Job drawing, mm, ordinate dimensions from the low corner. One solid piece. Give positions to 0.01 mm unless a question says otherwise; leave off trailing zeros. Loops run counter-clockwise (first coordinate to the right, second up) from the corner with the lowest first, then second, coordinate; pieces in that order, holes last. Notation, with made-up numbers: (87.25, 54) - (96.25, 54) arc R34 ccw to (96.25, 93) - close; hole circle Ø11 at (25.5, 38). An arc over 180 degrees is marked (long way). Use a Markdown table: item, result.
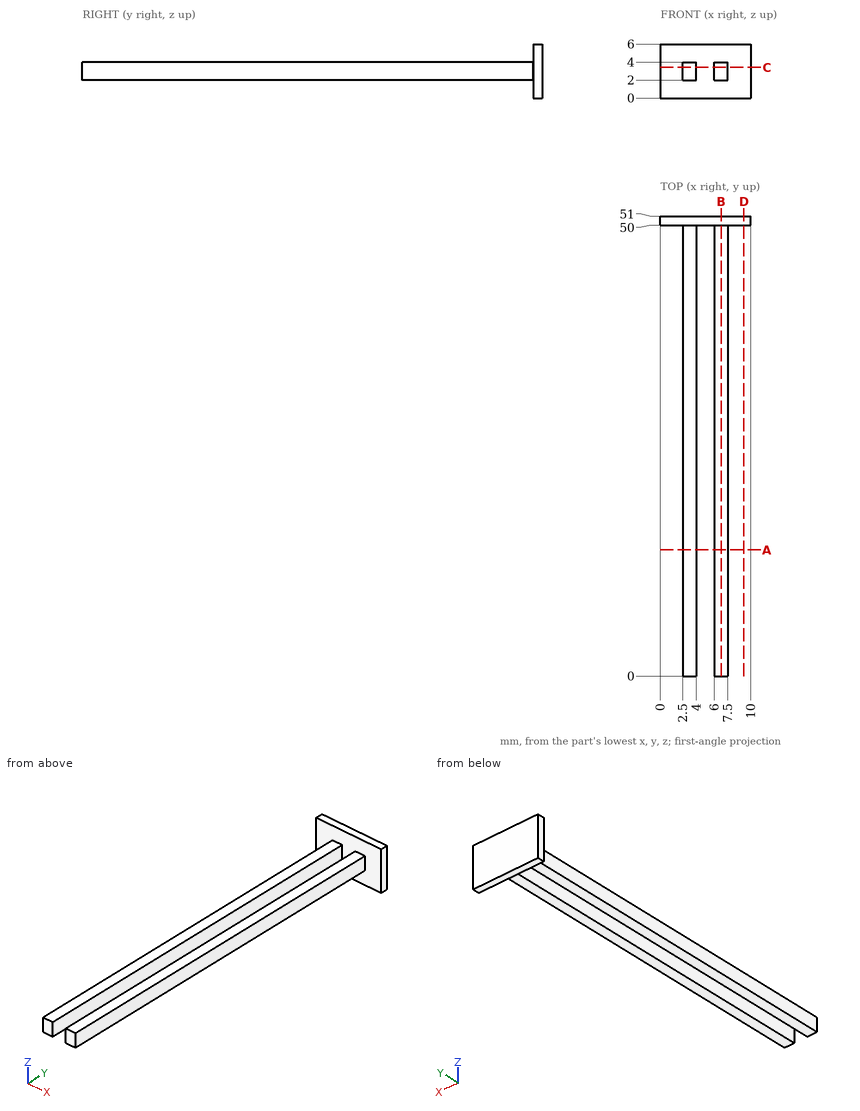
(1) Slice it at A-A, the plane y = 14. Write the cut outline in (x, z).
Computed:
| item | result |
|---|---|
| outline | (2.5, 2) - (4, 2) - (4, 4) - (2.5, 4) - close; (6, 2) - (7.5, 2) - (7.5, 4) - (6, 4) - close |
(2) Slice it at C-C, the plane z = 3.4. Write the cut outline in (x, y), plus the area to 3 significant figures.
Computed:
| item | result |
|---|---|
| outline | (0, 50) - (2.5, 50) - (2.5, 0) - (4, 0) - (4, 50) - (6, 50) - (6, 0) - (7.5, 0) - (7.5, 50) - (10, 50) - (10, 51) - (0, 51) - close |
| area | 160 mm² |
(3) Slice it at B-B, the plane x = 6.75. Write the cut outline in (y, z).
Computed:
| item | result |
|---|---|
| outline | (0, 2) - (50, 2) - (50, 0) - (51, 0) - (51, 6) - (50, 6) - (50, 4) - (0, 4) - close |
(4) Pin check, flat tips, straight feed: P1, Ø1, axis at x = 6.5, y = 17, coming from the +Z side; P2, Ø1.6, axis at y = 27.5, z = 3, coming from the +X side; P3, Ø1.6, axis at y = 28.5, z = 3, coming from the -X side. Stop position of each tip, or through.
Computed:
| item | result |
|---|---|
| P1 | z = 4 |
| P2 | x = 7.5 |
| P3 | x = 2.5 |
(5) Drill centre lines: probe 1 along X at (y, z) = (42, 3); probe 2 along Z at (x, y) = (2.75, 9); probe 3 along Y at (x, z) = (3.75, 5.45). Where is each one in solid material? Low to high. Write a range as [from, to].
Computed:
| item | result |
|---|---|
| probe 1 | [2.5, 4], [6, 7.5] |
| probe 2 | [2, 4] |
| probe 3 | [50, 51] |
(6) Slice it at D-D, the plane x = 9.25. Write the cut outline in (y, z), plus the area to 3 significant figures.
Computed:
| item | result |
|---|---|
| outline | (50, 0) - (51, 0) - (51, 6) - (50, 6) - close |
| area | 6.00 mm² |
